Read the model definition and answer for the solid it produces. Units are mm, in the model's axes. Face numbers are marked on the shaded views. A direction names the side the tool comes from. Coordinates: 2 decimals unless noted, no trailing zeros. Write each loop counter-clockwise with the first axis right and the second up, starting at its lowest first coordinate (ties: lowest second). Pieces come first, ordered by that corner, then holes. Notation, with made-up numbers: (82, 41.25) -> (86, 41.25) arc R26 ccw to (86, 68.25) -> close; hole circle Ø2 at (57.25, 57). An arc over 180 degrees is marked (long way). Answer as a JSON object with one key per item and string values. Group by question number.
(1) Flat-ended cylindrical pins translate along their axes: P1, Ø4, axis at x = -54.5, y = -15.5, coming from the -Z side; P2, Ø2.5, axis at x = 57.5, y = -25.5, coming from the -Z side; P3, Ø0.8, axis at y = -3, z = -2.5, coming from the -X side. Find the tip coordinate at first contact, or state that the pin passes through.
(2) Find section B-B (x = -3.5). Give the vertices of the cut face in (y, z), then the cut area to 3 significant figures.
(3) For a pull along Y with two mould halves and no side action, classify the marked faces 4 and 5 as +Y half, -Y half, draft (parallel to the pull), parting line (faces both ways), or undercut.
(4) Straight lines are drawn through the part: L1, parallel to Z at x = 4.5, y = 26.5; L2, parallel to Y at x = 34, z = 2.5; L3, parallel to Z at x = -42, y = 50. For each, find the intervals that lie inside material, in ascending order.
(5) Find section A-A (y = -39.5). Give the vertices of the cut face in (x, z).
(6) Which of the six approach directions +Z, -Z, +X, -X, +Y, -Y give full straight-line access (tool end or side, diameter ignored) to the marked faces 1, 2 and 3?
(7) Find section D-D (x = -43). Give the vertices of the cut face in (y, z), then the cut area to 3 significant figures.
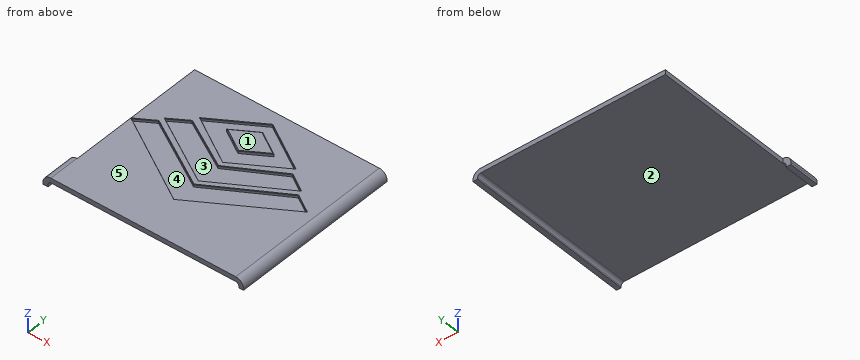
from build123d import *
from OCP.BRepFilletAPI import BRepFilletAPI_MakeChamfer

# Parameters (mm, degrees)
SKETCH1_W           = 129
SKETCH1_H           = 110
BOSS_EXTRUDE1_DEPTH = 3
SKETCH8_W           = 3
SKETCH8_H           = 110
BOSS_EXTRUDE5_DEPTH = 3
FILLET4_R           = 2
FILLET5_R           = 5
SKETCH9_W           = 1
SKETCH9_H           = 110
BOSS_EXTRUDE6_DEPTH = 2.5
BOSS_EXTRUDE7_DEPTH = 110
CUT_EXTRUDE3_DEPTH  = 1.75
CHAMFER3_SIZE       = 0.25
CHAMFER3_SIZE2      = 0.433012702
SKETCH14_W          = 3.26
SKETCH14_H          = 110
BOSS_EXTRUDE8_DEPTH = 3.5
FILLET6_R           = 2
FILLET7_R           = 5
CUT_EXTRUDE4_START  = -6.5
SKETCH17_W          = 5.25
SKETCH17_H          = 90
CUT_EXTRUDE4_DEPTH  = 6.5
SKETCH18_W          = 3
SKETCH18_H          = 3.302013378
CUT_EXTRUDE5_DEPTH  = 110


with BuildPart() as part:
    # Sketch1 → Boss-Extrude1 (new body)
    with BuildSketch(Plane.XY):
        with Locations((-5, 1)):
            Rectangle(SKETCH1_W, SKETCH1_H)
    extrude(amount=BOSS_EXTRUDE1_DEPTH)

    # Sketch8 → Boss-Extrude5 (add)
    with BuildSketch(Plane(origin=(0, 0, 0), x_dir=(-1, 0, 0), z_dir=(0, 0, -1))):
        with Locations((-58, 1)):
            Rectangle(SKETCH8_W, SKETCH8_H)
    extrude(amount=BOSS_EXTRUDE5_DEPTH)

    # Fillet4
    fillet4_edges = [part.edges().sort_by_distance(p)[0] for p in [
        (56.5, 1, 0),
    ]]
    fillet(fillet4_edges, radius=FILLET4_R)

    # Fillet5
    fillet5_edges = [part.edges().sort_by_distance(p)[0] for p in [
        (59.5, 1, 3),
    ]]
    fillet(fillet5_edges, radius=FILLET5_R)

    # Sketch9 → Boss-Extrude6 (add)
    with BuildSketch(Plane(origin=(0, 0, -3), x_dir=(-1, 0, 0), z_dir=(0, 0, -1))):
        with Locations((-58, 1)):
            Rectangle(SKETCH9_W, SKETCH9_H)
    extrude(amount=BOSS_EXTRUDE6_DEPTH)

    # Sketch10 → Boss-Extrude7 (add, through all)
    with BuildSketch(Plane(origin=(0, 56, 0), x_dir=(1, 0, 0), z_dir=(0, 1, 0))):
        Polygon((57.5, 5.5), (57, 3), (57.5, 3), align=None)
    extrude(amount=-BOSS_EXTRUDE7_DEPTH)

    # Sketch13 → Cut-Extrude3 (cut)
    # profile 1 of 3: a face of its own
    with BuildSketch(Plane.XY.offset(3)):
        Polygon((-7.5, 48), (-38.1126801, 29.056298749), (-7.5, 10.112597497), (23.1126801, 29.056298749), align=None)
        Polygon((-7.5, 40.5), (-22.80634005, 31.028149374), (-7.5, 21.556298749), (7.80634005, 31.028149374), align=None, mode=Mode.SUBTRACT)
    # profile 2 of 3: a face of its own
    with BuildSketch(Plane.XY.offset(3)):
        Polygon((-39.806973372, 24.905034542), (-51.197681844, 17.659224685), (-7.5, -8.637402503), (36.197681844, 17.659224685), (24.806973372, 24.905034542), (-7.5, 6.362597497), align=None)
    # profile 3 of 3: a face of its own
    with BuildSketch(Plane.XY.offset(3)):
        Polygon((-52.431392449, 14.281539595), (-63.876517147, 7.121992079), (-7.5, -27.387402503), (48.876517147, 7.121992079), (37.431392449, 14.281539595), (-7.5, -12.387402503), align=None)
    extrude(amount=-CUT_EXTRUDE3_DEPTH, mode=Mode.SUBTRACT)

    # Chamfer3: one chamfer whose edges measure the first distance from different faces: ONE call of the kernel's chamfer builder (chamfer() names one face for all edges)
    chamfer3_edges_1 = [part.edges().sort_by_distance(p)[0] for p in [
        (-23.653486686, 15.63381602, 3),
        (-45.502327608, 21.282129613, 3),
        (-29.348840922, 4.510911091, 3),
        (14.348840922, 4.510911091, 3),
        (30.502327608, 21.282129613, 3),
        (8.653486686, 15.63381602, 3),
        (-29.965696224, 0.947068546, 3),
        (-58.153954798, 10.701765837, 3),
        (-35.688258573, -10.132705212, 3),
        (20.688258573, -10.132705212, 3),
        (43.153954798, 10.701765837, 3),
        (14.965696224, 0.947068546, 3),
        (7.80634005, 38.528149374, 3),
        (-22.80634005, 38.528149374, 3),
        (-22.80634005, 19.584448123, 3),
        (7.80634005, 19.584448123, 3),
    ]]
    chamfer3_side_1 = [part.faces().sort_by_distance(p)[0] for p in [
        (-7.5, 54.34241139, 3),
    ]]
    chamfer3_edges_2 = [part.edges().sort_by_distance(p)[0] for p in [
        (0.153170025, 35.764074687, 3),
    ]]
    chamfer3_side_2 = [part.faces().sort_by_distance(p)[0] for p in [
        (0.153170025, 35.764074687, 2.125),
    ]]
    chamfer3_edges_3 = [part.edges().sort_by_distance(p)[0] for p in [
        (0.153170025, 26.292224061, 3),
    ]]
    chamfer3_side_3 = [part.faces().sort_by_distance(p)[0] for p in [
        (0.153170025, 26.292224061, 2.125),
    ]]
    chamfer3_edges_4 = [part.edges().sort_by_distance(p)[0] for p in [
        (-15.153170025, 26.292224061, 3),
    ]]
    chamfer3_side_4 = [part.faces().sort_by_distance(p)[0] for p in [
        (-15.153170025, 26.292224061, 2.125),
    ]]
    chamfer3_edges_5 = [part.edges().sort_by_distance(p)[0] for p in [
        (-15.153170025, 35.764074687, 3),
    ]]
    chamfer3_side_5 = [part.faces().sort_by_distance(p)[0] for p in [
        (-15.153170025, 35.764074687, 2.125),
    ]]
    chamfer3 = BRepFilletAPI_MakeChamfer(part.part.solid().wrapped)
    for e in chamfer3_edges_1:
        chamfer3.Add(CHAMFER3_SIZE, CHAMFER3_SIZE2, e.wrapped, chamfer3_side_1[0].wrapped)  # the first distance lies on this face
    for e in chamfer3_edges_2:
        chamfer3.Add(CHAMFER3_SIZE, CHAMFER3_SIZE2, e.wrapped, chamfer3_side_2[0].wrapped)  # the first distance lies on this face
    for e in chamfer3_edges_3:
        chamfer3.Add(CHAMFER3_SIZE, CHAMFER3_SIZE2, e.wrapped, chamfer3_side_3[0].wrapped)  # the first distance lies on this face
    for e in chamfer3_edges_4:
        chamfer3.Add(CHAMFER3_SIZE, CHAMFER3_SIZE2, e.wrapped, chamfer3_side_4[0].wrapped)  # the first distance lies on this face
    for e in chamfer3_edges_5:
        chamfer3.Add(CHAMFER3_SIZE, CHAMFER3_SIZE2, e.wrapped, chamfer3_side_5[0].wrapped)  # the first distance lies on this face
    add(Compound.cast(chamfer3.Shape()), mode=Mode.REPLACE)

    # Sketch14 → Boss-Extrude8 (add)
    with BuildSketch(Plane(origin=(0, 0, 0), x_dir=(-1, 0, 0), z_dir=(0, 0, -1))):
        with Locations((67.87, 1)):
            Rectangle(SKETCH14_W, SKETCH14_H)
    extrude(amount=BOSS_EXTRUDE8_DEPTH)

    # Fillet6
    fillet6_edges = [part.edges().sort_by_distance(p)[0] for p in [
        (-66.24, 1, 0),
    ]]
    fillet(fillet6_edges, radius=FILLET6_R)

    # Fillet7
    fillet7_edges = [part.edges().sort_by_distance(p)[0] for p in [
        (-69.5, 1, 3),
    ]]
    fillet(fillet7_edges, radius=FILLET7_R)

    # Sketch17 → Cut-Extrude4 (cut)
    with BuildSketch(Plane(origin=(0, 0, -3.5), x_dir=(-1, 0, 0), z_dir=(0, 0, -1)).offset(CUT_EXTRUDE4_START)):
        with Locations((66.875, 11)):
            Rectangle(SKETCH17_W, SKETCH17_H)
    extrude(amount=CUT_EXTRUDE4_DEPTH, mode=Mode.SUBTRACT)

    # Sketch18 → Cut-Extrude5 (cut)
    with BuildSketch(Plane(origin=(0, 56, 0), x_dir=(1, 0, 0), z_dir=(0, 1, 0))):
        with Locations((58, 4.651006689)):
            Rectangle(SKETCH18_W, SKETCH18_H)
    extrude(amount=-CUT_EXTRUDE5_DEPTH, mode=Mode.SUBTRACT)


solid = part.part
Results below:
{
 "1": {"P1": "stops at z = 0", "P2": "stops at z = -3", "P3": "stops at x = 56.5"},
 "2": {"outline": "(-54, 0) -> (56, 0) -> (56, 3) -> (45.82, 3) -> (45.52, 2.57) -> (45.52, 1.25) -> (38.02, 1.25) -> (38.02, 2.75) -> (37.52, 3) -> (24.54, 3) -> (24.03, 2.75) -> (24.03, 1.25) -> (12.59, 1.25) -> (12.59, 2.57) -> (12.29, 3) -> (8.95, 3) -> (8.66, 2.57) -> (8.66, 1.25) -> (-6.23, 1.25) -> (-6.23, 2.57) -> (-6.52, 3) -> (-9.72, 3) -> (-10.01, 2.57) -> (-10.01, 1.25) -> (-24.94, 1.25) -> (-24.94, 2.57) -> (-25.23, 3) -> (-54, 3) -> close", "area": "244 mm2"},
 "3": {"face 4": "undercut", "face 5": "draft"},
 "4": {"L1": "z = 0 to 1.25", "L2": "y = -54 to -1.98, 12.24 to 16.34, 19.06 to 56", "L3": "z = 0 to 3"},
 "5": {"outline": "(-69.5, -3.5) -> (-66.24, -3.5) -> (-66.24, -2) arc R2 cw to (-64.24, 0) -> (54.5, 0) arc R2 cw to (56.5, -2) -> (56.5, -3) -> (59.5, -3) -> (59.5, -2) arc R5 ccw to (54.5, 3) -> (-64.5, 3) arc R5 ccw to (-69.5, -2) -> close"},
 "6": {"face 1": "+Z, +X, -X, +Y, -Y", "face 2": "-Z, +Y, -Y", "face 3": "+Z"},
 "7": {"outline": "(-54, 0) -> (56, 0) -> (56, 3) -> (23.17, 3) -> (22.87, 2.57) -> (22.87, 1.25) -> (12.73, 1.25) -> (12.73, 2.57) -> (12.43, 3) -> (8.97, 3) -> (8.68, 2.57) -> (8.68, 1.25) -> (-5.66, 1.25) -> (-5.66, 2.57) -> (-5.95, 3) -> (-54, 3) -> close", "area": "287 mm2"}
}
